```python
from build123d import *

# Parameters (mm, degrees)
SKETCH1_R           = 10
BOSS_EXTRUDE1_DEPTH = 150
CUT_EXTRUDE1_START  = -20
CUT_EXTRUDE1_DEPTH  = 20
SKETCH3_3_R         = 1
CUT_EXTRUDE4_DEPTH  = 152.348108677
SKETCH7_R           = 1
CUT_EXTRUDE5_DEPTH  = 10
SKETCH8_R           = 5
CUT_EXTRUDE6_DEPTH  = 151.665191733


with BuildPart() as part:
    # Sketch1 → Boss-Extrude1 (new body)
    with BuildSketch(Plane.XY):
        Circle(SKETCH1_R)
    extrude(amount=BOSS_EXTRUDE1_DEPTH)

    # Sketch2 → Cut-Extrude1 (cut)
    with BuildSketch(Plane.XY.offset(150).offset(CUT_EXTRUDE1_START)):
        with BuildLine():
            ThreePointArc((6.614378278, 7.5), (0, 10), (-6.614378278, 7.5))
            Line((-6.614378278, 7.5), (6.614378278, 7.5))
        make_face()
        with BuildLine():
            Line((-6.614378278, -7.5), (-6.614378278, 7.5))
            ThreePointArc((-6.614378278, 7.5), (-10, 0), (-6.614378278, -7.5))
        make_face()
        with BuildLine():
            ThreePointArc((6.614378278, -7.5), (10, 0), (6.614378278, 7.5))
            Line((6.614378278, 7.5), (6.614378278, -7.5))
        make_face()
        with BuildLine():
            Line((6.614378278, -7.5), (-6.614378278, -7.5))
            ThreePointArc((-6.614378278, -7.5), (0, -10), (6.614378278, -7.5))
        make_face()
    extrude(amount=CUT_EXTRUDE1_DEPTH, mode=Mode.SUBTRACT)

    # Sketch3_3 → Cut-Extrude4 (cut, through all)
    with BuildSketch(Plane(origin=(0, 7.5, 0), x_dir=(1, 0, 0), z_dir=(0, 1, 0))):
        with Locations(Location((0.114378278, -145, 0), (0, 0, 270))):
            Circle(SKETCH3_3_R)
    extrude(amount=-CUT_EXTRUDE4_DEPTH, mode=Mode.SUBTRACT)

    # Sketch7 → Cut-Extrude5 (cut)
    with BuildSketch(Plane(origin=(0, 0, 0), x_dir=(-1, 0, 0), z_dir=(0, 0, -1))):
        with Locations((7.5, 0)):
            Circle(SKETCH7_R)
        with Locations((-7.5, 0)):
            Circle(SKETCH7_R)
    extrude(amount=-CUT_EXTRUDE5_DEPTH, mode=Mode.SUBTRACT)

    # Sketch8 → Cut-Extrude6 (cut, through all)
    with BuildSketch(Plane(origin=(0, 0, 0), x_dir=(-1, 0, 0), z_dir=(0, 0, -1))):
        Circle(SKETCH8_R)
    extrude(amount=-CUT_EXTRUDE6_DEPTH, mode=Mode.SUBTRACT)


solid = part.part
```
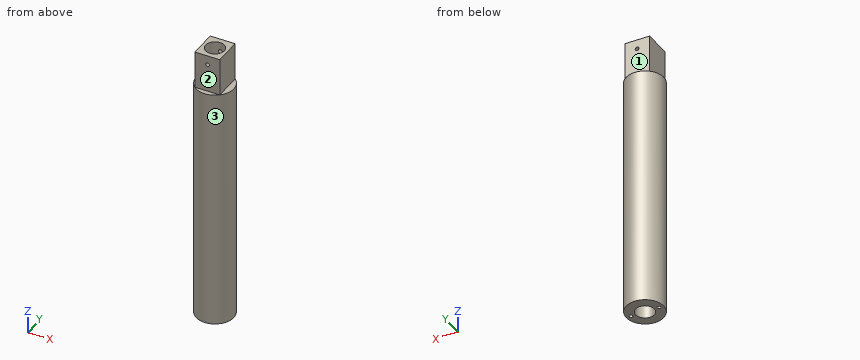
The listing builds one solid part. Answer for the finished solid, in the listing's coordinates (mm). Face numbers are marked on the shaded views. A direction names the side the tool comes from. Give positions to 0.01 mm unless a question says otherwise; leave off trailing zeros. Write each loop counter-clockwise with the first axis right and the second up, starting at its lowest first coordinate (ties: lowest second). Pieces come first, ordered by that corner, then holes. Notation, with made-up numbers: (-37.75, 11.5) -> (-21.75, 11.5) arc R24 cw to (-21.75, 30.5) -> close; hole circle Ø8 at (26.25, -15.75). An arc over 180 degrees is marked (long way). Write item = value, one per line. Start each with the question number.
1) Each of these flat-tipped pins is pushed along its axis until it touches: pin 1 (2 mm diameter, centred on y = -2.5, z = 117.5, fed in from +X); pin 2 (1.2 mm diameter, centred on x = -0.5, y = -8.5, fed in from +Z); pin 3 (4.5 mm diameter, centred on y = 0, z = 143, fed in from -X). Where does it stop, or does it pass through?
2) The part is cut by section B-B, the plane y = 3.5. Determine the outline of the cut face in (x, z).
3) Straight lines are drawn through the part: line 1 along Z through (x, y) = (0, 6.5); line 2 along Y through (x, z) = (-7.5, 5.5); line 3 along X through (y, z) = (6.4, 145). For each, find the intervals that lie inside material, in ascending order.
4) Which of the six approach directions +Z, -Z, +X, -X, +Y, -Y give full straight-line access (tool end or side, diameter ignored) to the marked faces 1, 2 and 3?
5) The part is cut by section C-C, the plane z = 113. Determine the outline of the cut face in (x, y).
6) The part is cut by section A-A, the plane x = 2.75. Determine the outline of the cut face in (y, z).
Solutions:
q1.pin_1 = 9.89
q1.pin_2 = 130
q1.pin_3 = -6.61
q2.outline = (-9.37, 0) -> (-3.57, 0) -> (-3.57, 150) -> (-6.61, 150) -> (-6.61, 130) -> (-9.37, 130) -> close; (3.57, 0) -> (9.37, 0) -> (9.37, 130) -> (6.61, 130) -> (6.61, 150) -> (3.57, 150) -> close
q3.line_1 = 0 to 144.01, 145.99 to 150
q3.line_2 = -6.61 to -1, 1 to 6.61
q3.line_3 = -6.61 to -0.89, 1.11 to 6.61
q4.face_1 = +Z, +X, -X, +Y
q4.face_2 = +Z, +X, -X, -Y
q4.face_3 = +Z, -Z
q5.outline = circle Ø20 at (0, 0); hole circle Ø10 at (0, 0)
q6.outline = (-9.61, 0) -> (-4.18, 0) -> (-4.18, 150) -> (-7.5, 150) -> (-7.5, 130) -> (-9.61, 130) -> close; (4.18, 0) -> (9.61, 0) -> (9.61, 130) -> (7.5, 130) -> (7.5, 150) -> (4.18, 150) -> close
